Part model, mm, in its own coordinate system. A direction names the side the tool comes from. Round coordinates to 2 decimals unless told otherwise and drop trailing zeros. Order: outer loops, then holes, each group sorted by start corner. A loop starts at its lowest first (then second) coordinate and runs counter-clockwise, first axis right, second up. Notation, with made-up numbers: (33, 4) -> (68, 4) arc R17 cw to (68, 25) -> close; hole circle Ø4 at (69.5, 56.25). An arc over 180 degrees is marked (long way). Return JSON: item names as keys, results as strings. Group by question number.
from build123d import *

# Parameters (mm, degrees)
F0_W     = 25.4
F0_H     = 25.4
F0_W_2   = 22.225
F0_H_2   = 22.225
F1_DEPTH = 685.8
F2_W     = 22.225
F2_H     = 22.225
F3_DEPTH = 12.7
F4_R     = 3.175
F5_DEPTH = 1.5875
F6_R     = 2.15265
F7_DEPTH = 25.4


with BuildPart() as f1:
    # F0 (on Top) → F1 (new body)
    with BuildSketch(Plane.XY):
        Rectangle(F0_W, F0_H)
        Rectangle(F0_W_2, F0_H_2, mode=Mode.SUBTRACT)
    extrude(amount=F1_DEPTH)

    # F2 (on Front) → F3 (cut, through all)
    with BuildSketch(Plane.XZ):
        with Locations((0, 342.9)):
            Rectangle(F2_W, F2_H)
    extrude(amount=F3_DEPTH, mode=Mode.SUBTRACT)

    # F4 (on face) → F5 (cut, through all)
    with BuildSketch(Plane(origin=(0, 12.7, 0), x_dir=(-1, 0, 0), z_dir=(0, 1, 0))):
        with Locations((0, 342.9)):
            Circle(F4_R)
    extrude(amount=-F5_DEPTH, mode=Mode.SUBTRACT)

    # F6 (on face) → F7 (cut, through all)
    with BuildSketch(Plane(origin=(-12.7, 0, 0), x_dir=(0, -1, 0), z_dir=(-1, 0, 0))):
        with Locations((0, 12.7)):
            Circle(F6_R)
        with Locations((0, 63.5)):
            Circle(F6_R)
        with Locations((0, 673.1)):
            Circle(F6_R)
        with Locations((0, 622.3)):
            Circle(F6_R)
    extrude(amount=-F7_DEPTH, mode=Mode.SUBTRACT)


solid = f1.part
(1) Tool access for faces 5 (the flat face through (0, -11.112, 518)), 6 (the flat face through (-11.3, 0.1, 685.8)): list every direction of +Z, -Z, +X, -X, +Y, -Y with a clear straight run to the whole face (end or side of a thin tool).
(2) Probe L1, parallel to Z at x = -11.45, y = 0; L2, parallel to Y at x = 12.3, z = 673.1; L3, parallel to X at y = 10.75, z = 329.5. List the from-to ranges inside material, lowest first. Write a range as [from, to].
(3) Saw through at A-A, the plane z = 601. List the corners of the cut face in (x, y).
(4) Pin check, flat tip, straight feed: P1, Ø8.5, axis at x = 0, z = 342.9, coming from the -Y side. Stop position of the tip, or through.
(5) Saw through at B-B, the plane y = 6.5. List the corners of the cut face in (x, z).
(6) Mould opens along X. For faces 1 (the flat face through (12.7, 0, 338)), 2 (the flat face through (-11.3, 0.1, 0)), 3 (the flat face through (-11.112, -1, 338)), 4 (the flat face through (-12.7, 0, 338)) say: pulls with the +X half, pulls with the -X half, needs draft (parallel to the pull), parting line crosses it, or undercut.
Results are:
{
 "1": {"face 5": "+Z, -Z", "face 6": "+Z, +X, -X, +Y, -Y"},
 "2": {"L1": "z = [0, 10.55], [14.85, 61.35], [65.65, 620.15], [624.45, 670.95], [675.25, 685.8]", "L2": "y = [-12.7, -2.15], [2.15, 12.7]", "L3": "x = [-12.7, -11.11], [11.11, 12.7]"},
 "3": {"outline": "(-12.7, -12.7) -> (12.7, -12.7) -> (12.7, 12.7) -> (-12.7, 12.7) -> close; hole (-11.11, -11.11) -> (11.11, -11.11) -> (11.11, 11.11) -> (-11.11, 11.11) -> close"},
 "4": {"P1": "stops at y = 11.11"},
 "5": {"outline": "(-12.7, 0) -> (-11.11, 0) -> (-11.11, 685.8) -> (-12.7, 685.8) -> close; (11.11, 0) -> (12.7, 0) -> (12.7, 685.8) -> (11.11, 685.8) -> close"},
 "6": {"face 1": "pulls with the +X half", "face 2": "needs draft", "face 3": "undercut", "face 4": "pulls with the -X half"}
}
